For this review, take the finished solid that the model builds, in its own axes (mm). A direction names the side the tool comes from. Coordinates: 2 decimals unless noted, no trailing zeros. Write each loop counter-clockwise with the first axis right and the second up, starting at its lowest first coordinate (ties: lowest second). Pieces come first, ordered by that corner, then holes. Notation, with made-up numbers: (-5.5, 66) -> (9.5, 66) arc R11 ccw to (9.5, 75) -> close; hole circle Ø2 at (85, 9). An arc over 180 degrees is marked (long way). Put each result on its own line as item: value. Start each with the question number.
Item 1: For faces 1 (the flat face through (-30, -90, 20)), 2 (the flat face through (-60, -70, 20)), 3 (the flat face through (-41, -25, 30)), list the 3-axis set-ups (+Z, -Z, +X, -X, +Y, -Y) from which the entire face can be reached by the end or side of a thin tool; tool diameter is ignored.
Item 2: Consider section A-A on x = -25.5. Give the boundary of the cut face in (y, z).
Item 3: To check wall thickness, follow L1, parallel to Z at x = -10.5, y = -47.5; L2, parallel to Y at x = -55, z = 29; L3, parallel to X at y = -81, z = 36. State the ranges of each line that lie inside material, in increasing order.
Item 4: The part is to be moulded in two halves that separate along Y. For faces 4 (the flat face through (-40.6, -48.7, 28.8)), 5 (the flat face through (-70, -50, 14)), 6 (the flat face through (-30, -50, 34)), 7 (the flat face through (-1.3, -25.3, 28.8)), say which applies: +Y half, -Y half, draft (parallel to the pull), parting line (faces both ways), or undercut.
Item 5: Consider section B-B on z = 15. Give the boundary of the cut face in (x, y), and give its area (3 significant figures).
Item 6: Consider section C-C on y = -28. Give the boundary of the cut face in (x, z).
Item 7: Consider section D-D on y = -54. Give the boundary of the cut face in (x, z).
Item 8: Insertion check: P1, Ø12, axis at y = -63.5, z = 20, coming from the -X side; P2, Ø22, axis at x = -73.5, z = 13, coming from the -Y side; P3, Ø22.5, axis at x = -55.5, y = -33, coming from the +Z side; P4, Ø14, axis at x = -31.5, z = 33, coming from the +Y side. Each pin has a flat end and moves straight along its axis. Give the tip position at first contact, or say it passes through.
```python
from build123d import *

# Parameters (mm, degrees)
F0_W     = 80
F0_H     = 50
F1_DEPTH = 30
F2_SIZE  = 2.5
F3_W     = 60
F3_H     = 40
F4_DEPTH = 40


with BuildPart() as f1:
    # F0 (on Top) → F1 (new body)
    with BuildSketch(Plane.XY):
        with Locations((-40, -25)):
            Rectangle(F0_W, F0_H)
    extrude(amount=F1_DEPTH)

    # F2
    f2_edges = [f1.edges().sort_by_distance(p)[0] for p in [
        (0, -25, 30),
        (-40, 0, 30),
        (-80, -25, 30),
        (-40, -50, 30),
    ]]
    chamfer(f2_edges, length=F2_SIZE)

    # F3 (on face) → F4 (join)
    with BuildSketch(Plane.XZ.offset(50)):
        with Locations((-30, 20)):
            Rectangle(F3_W, F3_H)
    extrude(amount=F4_DEPTH)


solid = f1.part
```
Return value:
1. face 1: +Z, -Z, +X, -X, -Y
1. face 2: +Z, -Z, -X, -Y
1. face 3: +Z, +X, -X, +Y
2. outline: (-90, 0) -> (0, 0) -> (0, 27.5) -> (-2.5, 30) -> (-47.5, 30) -> (-50, 27.5) -> (-50, 40) -> (-90, 40) -> close
3. L1: 0 to 30
3. L2: -90 to -50, -48.5 to -1.5
3. L3: -60 to 0
4. face 4: undercut
4. face 5: -Y half
4. face 6: undercut
4. face 7: draft
5. outline: (-80, -50) -> (-60, -50) -> (-60, -90) -> (0, -90) -> (0, 0) -> (-80, 0) -> close
5. area: 6,400 mm^2
6. outline: (-80, 0) -> (0, 0) -> (0, 27.5) -> (-2.5, 30) -> (-77.5, 30) -> (-80, 27.5) -> close
7. outline: (-60, 0) -> (0, 0) -> (0, 40) -> (-60, 40) -> close
8. P1: x = -60
8. P2: y = -50
8. P3: z = 30
8. P4: y = 0
